Work out the finished part from the listing and answer in its coordinate system (mm). Face numbers are marked on the shaded views. Give positions to 0.01 mm unless a question says otherwise; leave off trailing zeros. Use one line per item in the form item = value. Start each with the question number.
from build123d import *

# Parameters (mm, degrees)
FILLET1_R = 8
FILLET2_R = 8


with BuildPart() as part:
    # Sketch1 → Revolve1 (revolve)
    with BuildSketch(Plane.XY):
        Polygon((-10, 40), (10, 40), (7.355095289, 55), (-7.355095289, 55), align=None)
    revolve(axis=Axis((0, 0, 0), (1, 0, 0)))

    # Fillet1
    fillet1_edges = [part.edges().sort_by_distance(p)[0] for p in [
        (7.355095289, -55, 0),
    ]]
    fillet(fillet1_edges, radius=FILLET1_R)

    # Fillet2
    fillet2_edges = [part.edges().sort_by_distance(p)[0] for p in [
        (-7.355095289, -55, 0),
    ]]
    fillet(fillet2_edges, radius=FILLET2_R)


solid = part.part
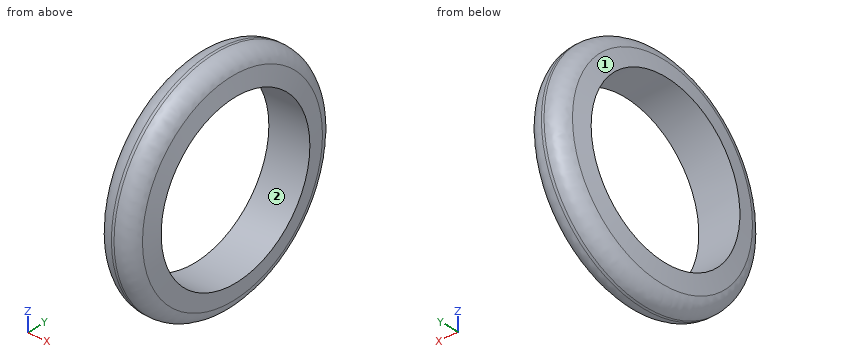
1) Flat-ended cylindrical pins translate along their axes: pin 1 Ø4 at (x, z) = (-2, 34) entering from +Y; pin 2 Ø5 at (x, z) = (2, -8) entering from +Y; pin 3 Ø2 at (y, z) = (35.5, 25.5) entering from -X. Find the tip coordinate at first contact, or state that the pin passes through.
2) Find the intervals of material crossed by probe 1 along Z at (x, y) = (0.5, 0); probe 2 along Z at (x, y) = (1, 33); probe 3 along Y at (x, z) = (4.5, 22.5), in increasing order.
3) Determine the mould class of the marked faces 1 and 2 for opening direction Z: released by +Z, released by -Z, zero draft, split by the parting line, or undercut.
Answer sheet:
q1.pin_1 = 44.63
q1.pin_2 = 54.69
q1.pin_3 = -9.52
q2.probe_1 = -55 to -40, 40 to 55
q2.probe_2 = -43.99 to -22.61, 22.61 to 43.99
q2.probe_3 = -49.1 to -33.07, 33.07 to 49.1
q3.face_1 = split by the parting line
q3.face_2 = undercut
